from build123d import *

# Parameters (mm, degrees)
EXTRUDE_1_DEPTH     = 5
CUT_EXTRUDE_1_REACH = 12.349
SKETCH_2_R          = 5


with BuildPart() as part:
    # 草图1 → 凸台-拉伸1 (new body)
    with BuildSketch(Plane(origin=(0, 0, 0), x_dir=(1, 0, 0), z_dir=(0, 1, 0))):
        Polygon((-6.47832956, 0), (6.47832956, 0), (3.5, -6.334789107), (-3.5, -6.334789107), align=None)
        Polygon((-6.47832956, 0), (-3.5, 6.334789107), (3.5, 6.334789107), (6.47832956, 0), align=None)
    extrude(amount=EXTRUDE_1_DEPTH)

    # 草图2 → 切除-拉伸1 (cut, up to next)
    with BuildSketch(Plane(origin=(0, 5, 0), x_dir=(1, 0, 0), z_dir=(0, 1, 0)), mode=Mode.PRIVATE) as cut_extrude_1_sk1:
        with Locations(Location((0, 0, 0), (0, 0, 270))):
            Circle(SKETCH_2_R)
    cut_extrude_1_tool1 = extrude(cut_extrude_1_sk1.sketch, amount=-CUT_EXTRUDE_1_REACH, mode=Mode.PRIVATE) & part.part
    add(cut_extrude_1_tool1.solids().sort_by_distance((0, 5, 0))[0], mode=Mode.SUBTRACT)


solid = part.part
Geometry: final body of the model. Coordinates: model frame, mm. Round coordinates to 2 decimals unless told otherwise and drop trailing zeros. Order: outer loops, then holes, each group sorted by start corner. A loop starts at its lowest first (then second) coordinate and runs counter-clockwise, first axis right, second up. Notation, with made-up numbers: (16, -35) - (51, -35) arc R20 ccw to (51, -12) - close; hole circle Ø4 at (57.25, -4.75). An arc over 180 degrees is marked (long way). Write each question's results on one line, items separated by ' | '.
Item 1: Section A-A, the plane x = 0. Return the cut outline in (y, z), and give its area (3 significant figures).
Completed:
outline: (0, -6.33) - (5, -6.33) - (5, -5) - (0, -5) - close; (0, 5) - (5, 5) - (5, 6.33) - (0, 6.33) - close | area: 13.3 mm^2
Item 2: Mould query, pull axis Z, two halves, no side actions, for faces 1 (the cylindrical face through (-4.88, 2.54, -1.08)), 2 (the flat face through (2, 0, 5)), 3 (the flat face through (0, 2, 6.335)). Classes: pulls with the +Z half, pulls with the -Z half, needs draft (parallel to the pull), parting line crosses it, or undercut.
Completed:
face 1: undercut | face 2: needs draft | face 3: pulls with the +Z half
Item 3: First-contact query: pin 1 Ø1.5 at (y, z) = (1, -4.5) entering from +X. Flat tip, straight axial feed; report the tip coordinate or a pass-through.
Completed:
pin 1: x = 4.72
Item 4: Material intervals for line 1 along Z through (x, y) = (-2, 4.15); line 2 along Z through (x, y) = (4, 3.15); line 3 along X through (y, z) = (1.15, -0.5), sorted ascending. Write a range as [from, to].
Completed:
line 1: [-6.33, -4.58], [4.58, 6.33] | line 2: [-5.27, -3], [3, 5.27] | line 3: [-6.24, -4.97], [4.97, 6.24]
Item 5: Section C-C, the plane z = -3. Return the cut outline in (x, y), and give its area (3 significant figures).
Completed:
outline: (-5.07, 0) - (-4, 0) - (-4, 5) - (-5.07, 5) - close; (4, 0) - (5.07, 0) - (5.07, 5) - (4, 5) - close | area: 10.7 mm^2
Item 6: Section B-B, the plane y = 0.8. Return the cut outline in (x, z).
Completed:
outline: (-6.48, 0) - (-3.5, -6.33) - (3.5, -6.33) - (6.48, 0) - (3.5, 6.33) - (-3.5, 6.33) - close; hole circle Ø10 at (0, 0)
